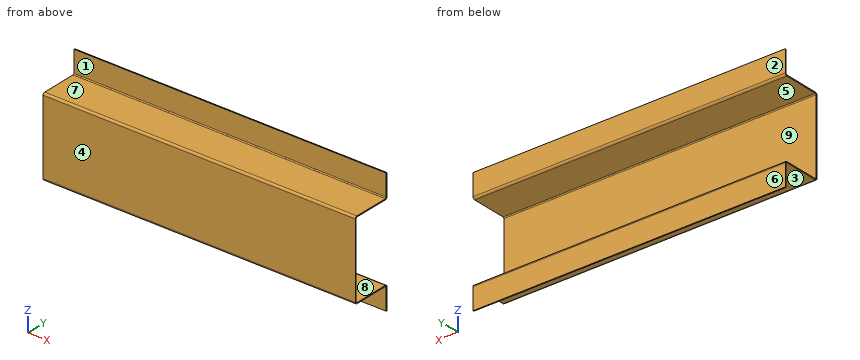
Autodesk Inventor part; units mm, degrees
ref_plane "YZ Plane" through (0, 0, 0) normal (1, 0, 0) x (0, 1, 0)
ref_plane "XZ Plane" through (0, 0, 0) normal (0, 1, 0) x (-1, 0, 0)
ref_plane "XY Plane" through (0, 0, 0) normal (0, 0, 1) x (1, 0, 0)
sketch "Sketch1" plane through (0, 0, 0) normal (0, 1, 0) x (-1, 0, 0)
  line L0 (254, 63.5) -> (-254, 63.5)
  line L1 (-254, 63.5) -> (-254, -63.5)
  line L2 (-254, -63.5) -> (254, -63.5)
  line L3 (254, -63.5) -> (254, 63.5)
  line L4 (254, 63.5) -> (-254, -63.5) construction
  line L5 (-254, 63.5) -> (254, -63.5) construction
  point P0 (0, 0)
  dimension "d0" = 508
  dimension "d1" = 127
extrude "Extrusion1" add sketch "Sketch1" along normal blind 1.5875
sketch "Sketch2" plane through (254, 0, 61.9125) normal (0, 0, 1) x (1, 0, 0)
  line L0 (-508, 0) -> (0, 0)
  line L1 (0, 0) -> (0, 63.5)
  line L2 (0, 63.5) -> (-508, 63.5)
  line L3 (-508, 63.5) -> (-508, 0)
edge flange "Flange1" height 63.5 angle 90 thickness 1.5875 bend radius 1.5875 thickness toward (0, 0, 1) relief straight relief width 1.5875 relief depth 0.7937 edges at (0, 1.5875, 63.5) wall of the first edge with corners at (-254, 0, 61.9125) (254, 0, 61.9125) (254, 63.5, 61.9125) (-254, 63.5, 61.9125)
bend "Bend1"
corner "Corner1"
sketch "Sketch3" plane through (-254, 61.9125, 61.9125) normal (0, 1, 0) x (-1, 0, 0)
  line L0 (-508, 0) -> (0, 0)
  line L1 (0, 0) -> (0, 38.1)
  line L2 (0, 38.1) -> (-508, 38.1)
  line L3 (-508, 38.1) -> (-508, 0)
edge flange "Flange2" height 38.1 angle 90 thickness 1.5875 bend radius 1.5875 thickness toward (0, 1, 0) relief straight relief width 1.5875 relief depth 0.7937 edges at (0, 63.5, 63.5) wall of the first edge with corners at (254, 61.9125, 61.9125) (-254, 61.9125, 61.9125) (-254, 61.9125, 100.0125) (254, 61.9125, 100.0125)
bend "Bend2"
corner "Corner2"
sketch "Sketch4" plane through (-254, 0, -61.9125) normal (0, 0, -1) x (-1, 0, 0)
  line L0 (-508, 0) -> (0, 0)
  line L1 (0, 0) -> (0, 63.5)
  line L2 (0, 63.5) -> (-508, 63.5)
  line L3 (-508, 63.5) -> (-508, 0)
edge flange "Flange3" height 63.5 angle 90 thickness 1.5875 bend radius 1.5875 thickness toward (0, 0, -1) relief straight relief width 1.5875 relief depth 0.7937 edges at (0, 1.5875, -63.5) wall of the first edge with corners at (254, 0, -61.9125) (-254, 0, -61.9125) (-254, 63.5, -61.9125) (254, 63.5, -61.9125)
bend "Bend3"
corner "Corner3"
sketch "Sketch5" plane through (254, 61.9125, -61.9125) normal (0, 1, 0) x (-1, 0, 0)
  line L0 (508, 0) -> (0, 0)
  line L1 (0, 0) -> (0, -38.1)
  line L2 (0, -38.1) -> (508, -38.1)
  line L3 (508, -38.1) -> (508, 0)
edge flange "Flange4" height 38.1 angle 90 thickness 1.5875 bend radius 1.5875 thickness toward (0, 1, 0) relief straight relief width 1.5875 relief depth 0.7937 edges at (0, 63.5, -63.5) wall of the first edge with corners at (-254, 61.9125, -61.9125) (254, 61.9125, -61.9125) (254, 61.9125, -100.0125) (-254, 61.9125, -100.0125)
bend "Bend4"
corner "Corner4"
equation "\"d4\" = Thickness"
equation "\"d5\" = BendReliefWidth"
equation "\"d6\" = BendReliefDepth"
equation "\"d7\" = MinimumRemnant"
equation "\"d8\" = TransitionRadius"
equation "\"d11\" = BendRadius"
equation "\"d12\" = CornerReliefSize"
equation "\"d13\" = GapSize"
equation "\"d14\" = JacobiRadiusSize"
equation "\"d15\" = BendReliefWidth"
equation "\"d16\" = BendReliefDepth"
equation "\"d17\" = MinimumRemnant"
equation "\"d18\" = TransitionRadius"
equation "\"d21\" = BendRadius"
equation "\"d22\" = CornerReliefSize"
equation "\"d23\" = GapSize"
equation "\"d24\" = JacobiRadiusSize"
equation "\"d25\" = BendReliefWidth"
equation "\"d26\" = BendReliefDepth"
equation "\"d27\" = MinimumRemnant"
equation "\"d28\" = TransitionRadius"
equation "\"d31\" = BendRadius"
equation "\"d32\" = CornerReliefSize"
equation "\"d33\" = GapSize"
equation "\"d34\" = JacobiRadiusSize"
equation "\"d35\" = BendReliefWidth"
equation "\"d36\" = BendReliefDepth"
equation "\"d37\" = MinimumRemnant"
equation "\"d38\" = TransitionRadius"
equation "\"d41\" = BendRadius"
equation "\"d42\" = CornerReliefSize"
equation "\"d43\" = GapSize"
equation "\"d44\" = JacobiRadiusSize"
equation "\"BendRadius\" = Thickness"
equation "\"BendReliefWidth\" = Thickness"
equation "\"BendReliefDepth\" = 0.5 * Thickness"
equation "\"CornerReliefSize\" = 4 * Thickness"
equation "\"MinimumRemnant\" = 2 * Thickness"
equation "\"TransitionRadius\" = BendRadius"
equation "\"JacobiRadiusSize\" = Thickness"
equation "\"GapSize\" = Thickness"
properties part number "Cubby Sheet Metal" material "Steel, Mild"
Model file for the job. Use its own axes, mm. Face numbers are marked on the shaded views. A direction names the side the tool comes from. Round coordinates to 2 decimals unless told otherwise and drop trailing zeros. Write each loop counter-clockwise with the first axis right and the second up, starting at its lowest first coordinate (ties: lowest second). Pieces come first, ordered by that corner, then holes. Notation, with made-up numbers: M 5.5,82.5 L 12.5,82.5 A26 ccw 12.5,99.5 Z; hole C -33,81.5 d8. An arc over 180 degrees is marked long. Put each result on its own line as item: value.
Item 1: Mould opens along Z. For the marked faces 6, 7, 8 and 9 say: +Z half, -Z half, draft (parallel to the pull), parting line (faces both ways), or undercut.
Responses:
face 6: draft
face 7: +Z half
face 8: undercut
face 9: undercut
Item 2: Cut at C-C (z = -20.5). List the corners of the cut face in (x, y), and give its area (3 significant figures).
Responses:
outline: M -254,0 L 254,0 L 254,1.59 L -254,1.59 Z
area: 806 mm²
Item 3: Tool access for the marked faces 1, 2, 3, 4 and 5: list every direction of +Z, -Z, +X, -X, +Y, -Y with a clear straight run to the whole face (end or side of a thin tool).
Responses:
face 1: +Z, +X, -X, -Y
face 2: +Z, -Z, +X, -X, +Y
face 3: -Z, +X, -X, -Y
face 4: +Z, -Z, +X, -X, -Y
face 5: +X, -X, +Y
Item 4: Flat gauge pins, fed straight in: P1, Ø17, axis at x = 118.5, y = 25, coming from the -Z side; P2, Ø10, axis at x = -133, y = 33.5, coming from the +Z side; P3, Ø17.5, axis at x = -40, z = -77.5, coming from the -Y side. Where does each tip first touch, or does it go through?
Responses:
P1: z = -63.5
P2: z = 63.5
P3: y = 61.91
Item 5: Probe L1, parallel to Z at x = 179, y = 54; L2, parallel to Y at x = 220, z = 31; L3, parallel to Y at x = 127, z = 73.5. List the from-to ranges inside material, lowest first. Write a range as from..to.
Responses:
L1: -63.5..-61.91, 61.91..63.5
L2: 0..1.59
L3: 61.91..63.5
Item 6: Cut at A-A (y = 9). List the corners of the cut face in (x, z).
Responses:
outline: M -254,-63.5 L 254,-63.5 L 254,-61.91 L -254,-61.91 Z; M -254,61.91 L 254,61.91 L 254,63.5 L -254,63.5 Z
